```python
from build123d import *

# Parameters (mm, degrees)
F0_W     = 76.2
F0_H     = 101.6
F0_R     = 1.778
F1_DEPTH = 11.43
F2_R     = 6.35
F3_R     = 5.08


with BuildPart() as f1:
    # F0 (on Right) → F1 (new body)
    with BuildSketch(Plane.YZ):
        with Locations((3.138589, -14.71612)):
            Rectangle(F0_W, F0_H)
        with Locations((-25.563411, -56.11812)):
            Circle(F0_R, mode=Mode.SUBTRACT)
        with Locations((31.840589, -56.11812)):
            Circle(F0_R, mode=Mode.SUBTRACT)
        with Locations((-25.563411, 26.68588)):
            Circle(F0_R, mode=Mode.SUBTRACT)
        with Locations((31.840589, 26.68588)):
            Circle(F0_R, mode=Mode.SUBTRACT)
    extrude(amount=F1_DEPTH)

    # F2
    f2_edges = [f1.edges().sort_by_distance(p)[0] for p in [
        (5.715, 41.238589, 36.08388),
        (5.715, 41.238589, -65.51612),
        (5.715, -34.961411, 36.08388),
        (5.715, -34.961411, -65.51612),
    ]]
    fillet(f2_edges, radius=F2_R)

    # F3
    f3_edges = [f1.edges().sort_by_distance(p)[0] for p in [
        (0, 3.138589, 36.08388),
    ]]
    fillet(f3_edges, radius=F3_R)


solid = f1.part
```
Here's how the part is built. I have some questions about the finished solid (model axes, mm). Coordinates: 2 decimals unless noted, no trailing zeros. Write each loop counter-clockwise with the first axis right and the second up, starting at its lowest first coordinate (ties: lowest second). Pieces come first, ordered by that corner, then holes. Notation, with made-up numbers: (36.5, 1) - (42.5, 1) arc R16 ccw to (42.5, 9) - close; hole circle Ø6 at (66, 27.5). An arc over 180 degrees is marked (long way). One line per item, written item: value.
1) Suppose I cut it at B-B on x = 2.75. State how many separate pieces and enclosed holes the cut face has, and give its area (3 significant figures).
Model answer:
separate pieces: 1
enclosed holes: 4
area: 7,470 mm²
2) We'd pull the mould along Z, two halves only. Please class faces 1 (the flat face through (8, 3, 36.084)), 2 (the cylindrical face through (5.63, -25.79, 28.45)), 3 (the flat face through (0, 3, -14)): pulls with the +Z half, pulls with the -Z half, needs draft (parallel to the pull), parting line crosses it, or undercut.
Model answer:
face 1: pulls with the +Z half
face 2: undercut
face 3: needs draft
3) Suppose I cut it at A-A on y = 32.5. Write out the boundary of the cut face in (x, z), and give its area (3 significant figures).
Model answer:
outline: (0, -60.44) arc R5.08 ccw to (5.08, -65.52) - (11.43, -65.52) - (11.43, -57.77) - (0, -57.77) - close; (0, -54.47) - (11.43, -54.47) - (11.43, 25.03) - (0, 25.03) - close; (0, 28.34) - (11.43, 28.34) - (11.43, 36.08) - (5.08, 36.08) arc R5.08 ccw to (0, 31) - close
area: 1,070 mm²
4) I need wall thicknesses on line 1 along Z through (x, y) = (2.25, 32); line 2 along Z through (x, y) = (1.25, 31); line 3 along Z through (x, y) = (5, 16). Which ranges of each line are inside material? Lowest first, please.
Model answer:
line 1: z = -64.65 to -57.89, -54.35 to 24.92, 28.46 to 35.22
line 2: z = -63.77 to -57.68, -54.55 to 25.12, 28.25 to 34.34
line 3: z = -65.52 to 36.08
5) I'm going to push flat-ended pins straight in: P1, Ø3, axis at y = -25.56, z = 26.69, coming from the -X side; P2, Ø1.5, axis at x = 3.5, z = 25.5, coming from the +Y side; P3, Ø5, axis at x = 1.5, z = -55.5, coming from the +Y side. Where does each tip first touch, or does it pass through?
Model answer:
P1: passes through
P2: stops at y = 41.17
P3: stops at y = 41.12
